from build123d import *

# Parameters (mm, degrees)
CROQUIS1_R              = 2.15
SALIENTE_EXTRUIR1_DEPTH = 318


with BuildPart() as part:
    # Croquis1 → Saliente-Extruir1 (new body)
    with BuildSketch(Plane.XY):
        Polygon((20, 4.95), (18.2, 6.75), (18.2, 4.4), (16.589949494, 4.4), (13.825, 7.164949494), (13.825, 12.835050506), (16.589949494, 15.6), (18.2, 15.6), (18.2, 13.25), (20, 15.05), (20, 20), (15.05, 20), (13.25, 18.2), (15.6, 18.2), (15.6, 16.589949494), (12.835050506, 13.825), (7.164949494, 13.825), (4.4, 16.589949494), (4.4, 18.2), (6.75, 18.2), (4.95, 20), (0, 20), (0, 15.05), (1.8, 13.25), (1.8, 15.6), (3.410050506, 15.6), (6.175, 12.835050506), (6.175, 7.164949494), (3.410050506, 4.4), (1.8, 4.4), (1.8, 6.75), (0, 4.95), (0, -4.95), (1.8, -6.75), (1.8, -4.4), (3.410050506, -4.4), (6.175, -7.164949494), (6.175, -12.835050506), (3.410050506, -15.6), (1.8, -15.6), (1.8, -13.25), (0, -15.05), (0, -20), (4.95, -20), (6.75, -18.2), (4.4, -18.2), (4.4, -16.589949494), (7.164949494, -13.825), (12.835050506, -13.825), (15.6, -16.589949494), (15.6, -18.2), (13.25, -18.2), (15.05, -20), (20, -20), (20, -15.05), (18.2, -13.25), (18.2, -15.6), (16.589949494, -15.6), (13.825, -12.835050506), (13.825, -7.164949494), (16.589949494, -4.4), (18.2, -4.4), (18.2, -6.75), (20, -4.95), align=None)
        with BuildLine():
            Line((1.8, -1.3), (1.8, 1.3))
            ThreePointArc((1.8, 1.3), (1.946446609, 1.653553391), (2.3, 1.8))
            Line((2.3, 1.8), (4.4, 1.8))
            Line((4.4, 1.8), (4.4, 3.410050506))
            Line((4.4, 3.410050506), (7.164949494, 6.175))
            Line((7.164949494, 6.175), (12.835050506, 6.175))
            Line((12.835050506, 6.175), (15.6, 3.410050506))
            Line((15.6, 3.410050506), (15.6, 1.8))
            Line((15.6, 1.8), (17.7, 1.8))
            ThreePointArc((17.7, 1.8), (18.053553391, 1.653553391), (18.2, 1.3))
            Line((18.2, 1.3), (18.2, -1.3))
            ThreePointArc((18.2, -1.3), (18.053553391, -1.653553391), (17.7, -1.8))
            Line((17.7, -1.8), (15.6, -1.8))
            Line((15.6, -1.8), (15.6, -3.410050506))
            Line((15.6, -3.410050506), (12.835050506, -6.175))
            Line((12.835050506, -6.175), (7.164949494, -6.175))
            Line((7.164949494, -6.175), (4.4, -3.410050506))
            Line((4.4, -3.410050506), (4.4, -1.8))
            Line((4.4, -1.8), (2.3, -1.8))
            ThreePointArc((2.3, -1.8), (1.946446609, -1.653553391), (1.8, -1.3))
        make_face(mode=Mode.SUBTRACT)
        with Locations(Location((10, -10, 0), (0, 0, 180))):
            Circle(CROQUIS1_R, mode=Mode.SUBTRACT)
        with Locations(Location((10, 10, 0), (0, 0, 180))):
            Circle(CROQUIS1_R, mode=Mode.SUBTRACT)
    extrude(amount=SALIENTE_EXTRUIR1_DEPTH)


solid = part.part
Can you work these out from the model? Positions are in its coordinate system, mm. A direction names the side the tool comes from. Give positions to 0.01 mm unless a question says otherwise; leave off trailing zeros. One line per item, written item: value.
1) I'm going to push flat-ended pins straight in: pin 1 (4 mm diameter, centred on x = 9, z = 119.5, fed in from -Y); pin 2 (3 mm diameter, centred on x = 11, z = 205.5, fed in from +Y) (3 decimals); pin 3 (4.5 mm diameter, centred on x = 9.5, z = 179.5, fed in from -Y) (3 decimals). Where does each tip first touch, or does it pass through?
Geometry check:
pin 1: stops at y = -13.99
pin 2: stops at y = 13.825
pin 3: stops at y = -13.825
2) Imagine slicing it at A-A on z = 158. Count the separate pieces of the cut face and the enclosed holes in it, and give its area (3 significant figures).
Geometry check:
separate pieces: 1
enclosed holes: 3
area: 292 mm²
3) Please list where these lines run through material, in increasing order: line 1 (Y direction, x = 1.25, z = 61); line 2 (Y direction, x = 10, z = 149) (3 decimals); line 3 (X direction, y = 2, z = 95).
Geometry check:
line 1: y = -20 to -13.8, -6.2 to 6.2, 13.8 to 20
line 2: y = -13.825 to -12.15, -7.85 to -6.175, 6.175 to 7.85, 12.15 to 13.825
line 3: x = 0 to 4.4, 15.6 to 20
4) Thinking about a two-plate mould opening in Y: for faces 1 (the face through (20, 17, 157)), 2 (the face through (17, -20, 157)), 3 (the face through (6.175, -10, 157)), 4 (the face through (10, 13.825, 157)), which applies, +Y half, -Y half, draft (parallel to the pull), parting line (faces both ways), or undercut?
Geometry check:
face 1: draft
face 2: -Y half
face 3: undercut
face 4: +Y half
5) On a 3-axis mill with a long thin cutter (end or side, diameter ignored), from which of +Z, -Z, +X, -X, +Y, -Y can I reach the whole of each face in a straight line? I mean faces 5 (the face through (13.825, -10, 157)), 6 (the face through (10, -13.825, 157)), 7 (the face through (10, -6.175, 157)), 8 (the face through (6.175, 10, 157)). Say none if no direction works.
Geometry check:
face 5: +Z, -Z, +X
face 6: +Z, -Z, -Y
face 7: +Z, -Z
face 8: +Z, -Z, -X
